Can you work these out from the model? Positions are in its coordinate system, mm. A direction names the side the tool comes from. Give positions to 0.01 mm unless a question says otherwise; leave off trailing zeros. Loops run counter-clockwise (first coordinate to the right, second up) from the corner with the lowest first, then second, coordinate; pieces in that order, holes last. Notation, with made-up numbers: (33.5, 51) -> (86.5, 51) arc R26 ccw to (86.5, 82) -> close; hole circle Ø8 at (-11, 68.5). An arc over 180 degrees is marked (long way). Use CSV: the item, a comma, the result in double quotes.
from build123d import *

# Parameters (mm, degrees)
F1_DEPTH    = 25
F2_T1_DEPTH = 32.0710678119


# Not quite as in the source:
# - a fillet or chamfer that OpenCascade refuses, or shapes differently, is made with other operations: its cross-section is extruded or revolved along the edge and cut away or added


with BuildPart() as f1:
    # F0 (on Front) → F1 (new body)
    with BuildSketch(Plane.XZ):
        with BuildLine():
            Line((9.5, 20), (0, 20))
            Line((0, 20), (0, 17.1773286244))
            Line((0, 17.1773286244), (8.65, 17.1773286244))
            Line((8.65, 17.1773286244), (8.65, 7.5421757065))
            ThreePointArc((8.65, 7.5421757065), (7.9600869661, 6.6679955593), (8.2, 5.5805156007))
            Line((8.2, 5.5805156007), (8.2, -20))
            Line((8.2, -20), (9.5, -20))
            Line((9.5, -20), (9.5, -4))
            Line((9.5, -4), (11, -4))
            Line((11, -4), (11, 0))
            Line((11, 0), (9.5, 0))
            Line((9.5, 0), (9.5, 15))
            Line((9.5, 15), (11, 15))
            Line((11, 15), (11, 19))
            Line((11, 19), (9.5, 19))
            Line((9.5, 19), (9.5, 20))
        make_face()
        with BuildLine():
            Line((0, 17.1773286244), (0, 20))
            Line((0, 20), (-9.5, 20))
            Line((-9.5, 20), (-9.5, 19))
            Line((-9.5, 19), (-11, 19))
            Line((-11, 19), (-11, 15))
            Line((-11, 15), (-9.5, 15))
            Line((-9.5, 15), (-9.5, 0))
            Line((-9.5, 0), (-11, 0))
            Line((-11, 0), (-11, -4))
            Line((-11, -4), (-9.5, -4))
            Line((-9.5, -4), (-9.5, -20))
            Line((-9.5, -20), (-8.2, -20))
            Line((-8.2, -20), (-8.2, 5.5805156007))
            ThreePointArc((-8.2, 5.5805156007), (-7.9600869661, 6.6679955593), (-8.65, 7.5421757065))
            Line((-8.65, 7.5421757065), (-8.65, 17.1773286244))
            Line((-8.65, 17.1773286244), (0, 17.1773286244))
        make_face()
    extrude(amount=F1_DEPTH)

    # F2: fillet of radius 1.5 on 2 edges, made by hand

    # F2_s2 → F2_t1 (cut)
    with BuildSketch(Plane.XZ.offset(-3.5355339059)):
        with BuildLine():
            ThreePointArc((-8.0857864376, 20), (-8.9518118414, 19.7247448714), (-9.5, 19))
            Line((-9.5, 19), (-9.5, 20))
            Line((-9.5, 20), (-8.0857864376, 20))
        make_face()
        with BuildLine():
            ThreePointArc((8.0857864376, 20), (8.9518118414, 19.7247448714), (9.5, 19))
            Line((9.5, 19), (9.5, 20))
            Line((9.5, 20), (8.0857864376, 20))
        make_face()
    extrude(amount=F2_T1_DEPTH, mode=Mode.SUBTRACT)


solid = f1.part
(1) Which directions (+Z, -Z, +X, -X, +Y, -Y) give clear straight access to the entire face, cutting with the end or side of a thin tool? Please do faces 1 (the face through (10, -12, 19)), 2 (the face through (-8.2, -12, -7)), 3 (the face through (10, -12, -4)).
Answer sheet:
face 1,"+Z, +X, +Y, -Y"
face 2,"-Z, +Y, -Y"
face 3,"-Z, +X, +Y, -Y"
(2) We'd pull the mould along Z, two halves only. Please class faces 4 (the face through (-8.2, 0, 6)), 5 (the face through (-10, -12, -4)), 6 (the face through (-9.5, -12, 8)), 7 (the face through (9.5, -12, 7)): released by +Z, released by -Z, zero draft, split by the parting line, or undercut.
Answer sheet:
face 4,"zero draft"
face 5,"released by -Z"
face 6,"undercut"
face 7,"undercut"
(3) If we section it at C-C, the plane z = -0.5: Write out the boundary of the cut face in (x, y).
Answer sheet:
outline,"(-11, -25) -> (-8.2, -25) -> (-8.2, 0) -> (-11, 0) -> close; (8.2, -25) -> (11, -25) -> (11, 0) -> (8.2, 0) -> close"
(4) If I drill on L1, parallel to X at y = -4.25, z = -11.5; L2, parallel to Z at x = -9.75, y = -6; L3, parallel to X at y = -10.25, z = 17, over which ranges is the centre line in solid material (lowest first)? Write a range as from..to.
Answer sheet:
L1,"x = -9.5..-8.2, 8.2..9.5"
L2,"z = -4..0, 15..19"
L3,"x = -11..-8.65, 8.65..11"
(5) Will these pins go through, and if not, where does the flat tip stop? pin 1 Ø8 at (x, z) = (1, 5.5) entering from -Y; pin 2 Ø0.8 at (x, y) = (10.5, -17.5) entering from -Z; pin 3 Ø12 at (y, z) = (-5, -13.5) entering from +X; pin 4 Ø3 at (y, z) = (-14, 10) entering from -X.
Answer sheet:
pin 1,"passes through"
pin 2,"stops at z = -4"
pin 3,"stops at x = 9.5"
pin 4,"stops at x = -9.5"
(6) If we section it at D-D, the plane x = -1.25: Write out the boundary of the cut face in (y, z).
Answer sheet:
outline,"(-25, 17.18) -> (0, 17.18) -> (0, 20) -> (-25, 20) -> close"
(7) If we section it at A-A, the plane z = -6: Write out the boundary of the cut face in (x, y), then the cut area to 3 significant figures.
Answer sheet:
outline,"(-9.5, -25) -> (-8.2, -25) -> (-8.2, 0) -> (-9.5, 0) -> close; (8.2, -25) -> (9.5, -25) -> (9.5, 0) -> (8.2, 0) -> close"
area,"65.0 mm2"
(8) If we section it at B-B, the plane y = -15: Write out the boundary of the cut face in (x, z), then the cut area to 3 significant figures.
Answer sheet:
outline,"(-11, -4) -> (-9.5, -4) -> (-9.5, -20) -> (-8.2, -20) -> (-8.2, 5.58) arc R1.3 ccw to (-8.65, 7.54) -> (-8.65, 17.18) -> (8.65, 17.18) -> (8.65, 7.54) arc R1.3 ccw to (8.2, 5.58) -> (8.2, -20) -> (9.5, -20) -> (9.5, -4) -> (11, -4) -> (11, 0) -> (9.5, 0) -> (9.5, 15) -> (11, 15) -> (11, 19) -> (9.5, 19) arc R1.5 ccw to (8.09, 20) -> (-8.09, 20) arc R1.5 ccw to (-9.5, 19) -> (-11, 19) -> (-11, 15) -> (-9.5, 15) -> (-9.5, 0) -> (-11, 0) -> close"
area,"165 mm2"
